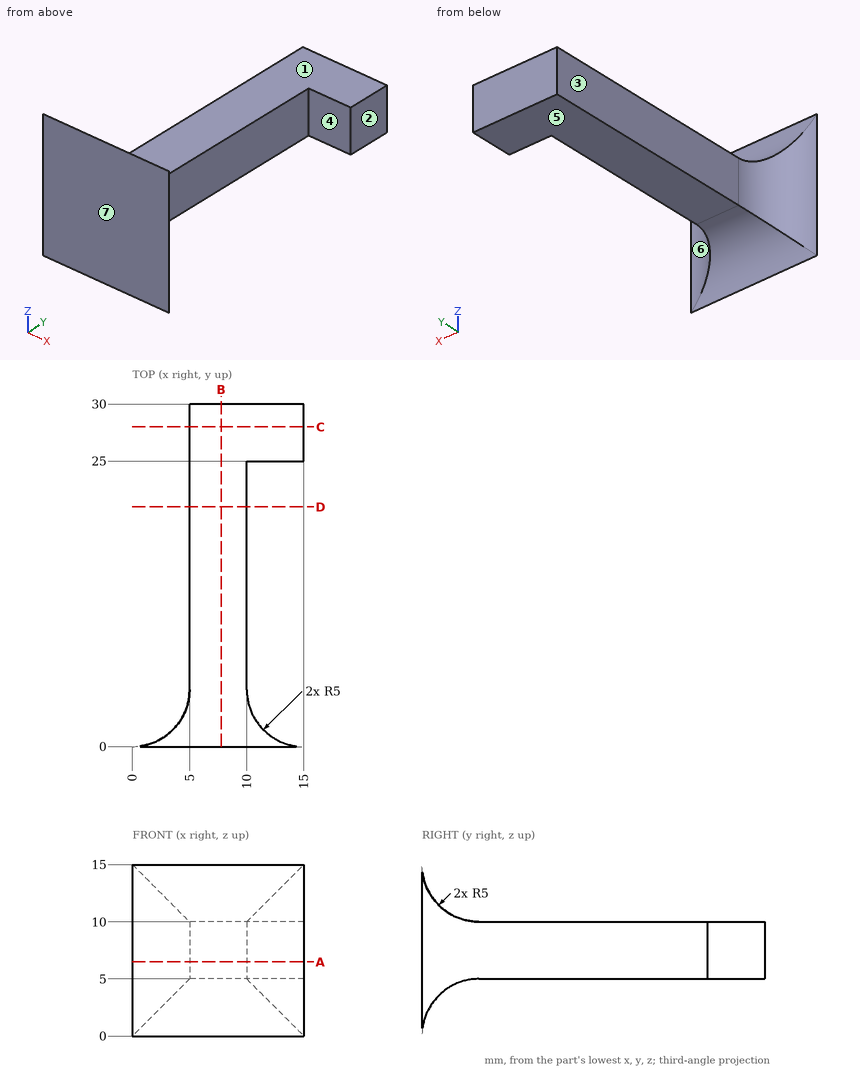
Here's the drawing with two shaded views (mm, measured from the low corner). I have some questions. A direction names the side the tool comes from. Give positions to 0.01 mm unless a question says otherwise; leave off trailing zeros. Order: outer loops, then holes, each group sorted by start corner. A loop starts at its lowest first (then second) coordinate and runs counter-clockwise, first axis right, second up. Notation, with made-up numbers: (-33, -1.5) -> (-24, -1.5) arc R26 cw to (-24, 28.5) -> close; hole circle Ø7 at (-18, 39). An arc over 180 degrees is marked (long way). One line per item, written item: value. Start each with the question number.
1. Imagine slicing it at C-C, the plane y = 28. List the corners of the cut face in (x, z) for me.
2. Imagine slicing it at D-D, the plane y = 21. List the corners of the cut face in (x, z) for me.
3. Imagine slicing it at B-B, the plane x = 7.75. List the corners of the cut face in (y, z) for me.
4. Imagine slicing it at A-A, the plane z = 6.5. List the corners of the cut face in (x, y) for me.
5. For the marked faces 1, 2, 3 and 4, which set-ups out of +Z, -Z, +X, -X, +Y, -Y let a thin tool reach every point of the face, with its end or its side?
6. I need wall thicknesses on probe 1 along Z at (x, y) = (9.25, 15.25); probe 2 along Y at (x, z) = (11.75, 6.5); probe 3 along Y at (x, z) = (12.25, 9) (1 decimal). Which ranges of each line are inside material? Lowest first, please. Write a range as from..to.
7. Will these pins go through, and if not, where does the flat tip stop? pin 1 Ø8 at (y, z) = (5.5, 9.5) entering from -X; pin 2 Ø1 at (x, y) = (5.5, 12.5) entering from +Z; pin 3 Ø4 at (x, z) = (11.5, 2) entering from +Y.
8. We'd pull the mould along Y, two halves only. Please class the marked faces 5, 6 and 7: released by +Y, released by -Y, zero draft, split by the parting line, or undercut.
Values follow:
1. outline: (5, 5) -> (15, 5) -> (15, 10) -> (5, 10) -> close
2. outline: (5, 5) -> (10, 5) -> (10, 10) -> (5, 10) -> close
3. outline: (0, 0) arc R5 cw to (5, 5) -> (30, 5) -> (30, 10) -> (5, 10) arc R5 cw to (0, 15) -> close
4. outline: (0, 0) -> (15, 0) arc R5 cw to (10, 5) -> (10, 25) -> (15, 25) -> (15, 30) -> (5, 30) -> (5, 5) arc R5 cw to start
5. face 1: +Z, +X, -X, +Y
5. face 2: +Z, -Z, +X, +Y, -Y
5. face 3: +Z, -Z, -X, +Y
5. face 4: +Z, -Z, +X
6. probe 1: z = 5..10
6. probe 2: y = 0..1.2, 25..30
6. probe 3: y = 0..0.8, 25..30
7. pin 1: stops at x = 3.57
7. pin 2: stops at z = 10
7. pin 3: stops at y = 1.93
8. face 5: zero draft
8. face 6: undercut
8. face 7: released by -Y
